```python
from build123d import *

# Parameters (mm, degrees)
EXTRUDE_1_DEPTH     = 64
SKETCH_2_W          = 73.114285432
SKETCH_2_H          = 69.176673978
SKETCH_2_R          = 31.5
CUT_EXTRUDE_2_DEPTH = 64
SKETCH_3_R          = 3.05
CUT_EXTRUDE_3_DEPTH = 64
SKETCH_4_R          = 1.55
CUT_EXTRUDE_4_DEPTH = 64


with BuildPart() as part:
    # 草图1 → 凸台-拉伸1 (new body)
    with BuildSketch(Plane(origin=(0, 0, 0), x_dir=(1, 0, 0), z_dir=(0, 1, 0))):
        with BuildLine():
            Line((-32, 0), (-7, 0))
            ThreePointArc((-7, 0), (-6.292893219, 0.292893219), (-6, 1))
            Line((-6, 1), (-6, 5))
            ThreePointArc((-6, 5), (-5.707106781, 5.707106781), (-5, 6))
            Line((-5, 6), (5, 6))
            ThreePointArc((5, 6), (5.707106781, 5.707106781), (6, 5))
            Line((6, 5), (6, 1))
            ThreePointArc((6, 1), (6.292893219, 0.292893219), (7, 0))
            Line((7, 0), (32, 0))
            Line((32, 0), (32, 2.5))
            Line((32, 2.5), (11, 2.5))
            ThreePointArc((11, 2.5), (10.292893219, 2.792893219), (10, 3.5))
            Line((10, 3.5), (10, 7.5))
            ThreePointArc((10, 7.5), (9.707106781, 8.207106781), (9, 8.5))
            Line((9, 8.5), (-9, 8.5))
            ThreePointArc((-9, 8.5), (-9.707106781, 8.207106781), (-10, 7.5))
            Line((-10, 7.5), (-10, 3.5))
            ThreePointArc((-10, 3.5), (-10.292893219, 2.792893219), (-11, 2.5))
            Line((-11, 2.5), (-32, 2.5))
            Line((-32, 2.5), (-32, 0))
        make_face()
    extrude(amount=EXTRUDE_1_DEPTH)

    # 草图2 → 切除-拉伸2 (cut)
    with BuildSketch(Plane.XY):
        with Locations((0, 32)):
            Rectangle(SKETCH_2_W, SKETCH_2_H)
        with Locations(Location((0, 32, 0), (0, 0, 290.438779576))):
            Circle(SKETCH_2_R, mode=Mode.SUBTRACT)
    extrude(amount=-CUT_EXTRUDE_2_DEPTH, mode=Mode.SUBTRACT)

    # 草图3 → 切除-拉伸3 (cut)
    with BuildSketch(Plane(origin=(0, 0, -2.5), x_dir=(-1, 0, 0), z_dir=(0, 0, -1))):
        with Locations((-17.67766953, 14.32233047)):
            Circle(SKETCH_3_R)
        with Locations((-17.67766953, 49.67766953)):
            Circle(SKETCH_3_R)
        with Locations((17.67766953, 49.67766953)):
            Circle(SKETCH_3_R)
        with Locations((17.67766953, 14.32233047)):
            Circle(SKETCH_3_R)
    extrude(amount=-CUT_EXTRUDE_3_DEPTH, mode=Mode.SUBTRACT)

    # 草图4 → 切除-拉伸4 (cut)
    with BuildSketch(Plane(origin=(0, 0, -8.5), x_dir=(-1, 0, 0), z_dir=(0, 0, -1))):
        with Locations((0, 54.5)):
            Circle(SKETCH_4_R)
        with Locations((0, 9.5)):
            Circle(SKETCH_4_R)
    extrude(amount=-CUT_EXTRUDE_4_DEPTH, mode=Mode.SUBTRACT)


solid = part.part
```
CAD build for the part. Positions are in the model's coordinates, mm. A direction names the side the tool comes from. Coordinates: 2 decimals unless noted, no trailing zeros. Order: outer loops, then holes, each group sorted by start corner. A loop starts at its lowest first (then second) coordinate and runs counter-clockwise, first axis right, second up. Notation, with made-up numbers: (29, -20) - (88, -20) arc R22 ccw to (88, 19) - close; hole circle Ø10 at (5.25, 63). An arc over 180 degrees is marked (long way). Use a Markdown table: item, result. Add a question column.
(1) Pull direction X, two halves, no side cores. Call faces 6 (the face through (-17.02, 46.7, -1.27)), 7 (the face through (-10, 32, -6)), 8 (the face through (-9.692, 61.972, -2.302)): +X half, -X half, draft (parallel to the pull), parting line (faces both ways), or undercut.
(2) Which spindle directions (+Z, -Z, +X, -X, +Y, -Y) get a long thin tool onto all of the face, cutting with end or side? Do faces 1 (the face through (6, 32, -3)), 2 (the face through (0, 32, -8.5)), 3 (the face through (10, 32, -5)), 4 (the face through (-19, 32, -2.5)), 5 (the face through (18.34, 46.7, -1.27)). Say none if no direction does.
(3) Drill centre lines: line 1 along Y through (x, z) = (0, -7.1); line 2 along X through (y, z) = (43, -5); line 3 along Y through (x, z) = (-18, -1.5). Where is each one in solid material? Low to high. Write a range as [from, to].
(4) Saw through at D-D (y = 9.5). Give the cut face in (x, z).
(5) Saw through at A-A (x = 0). Give the cut face in (y, z).
(6) Saw through at C-C (z = -6.75). Give the cut face in (x, y), then the cut area to 3 significant figures.
(7) Saw through at B-B (y = 32). Give the cut face in (x, z), then the cut area to 4 significant figures.
(8) Flat gauge pins, fed straight in: pin 1 (1.2 mm diameter, centred on y = 36, z = -3.5, fed in from -X); pin 2 (8 mm diameter, centred on x = -1.5, y = 23, fed in from +Z); pin 3 (2.5 mm diameter, centred on x = 0, y = 54.5, fed in from +Z); pin 4 (2 mm diameter, centred on y = 21, z = -6, fed in from +X). Where does each tip first touch, or does it go through?
Solved:
| question | item | result |
|---|---|---|
| 1 | face 6 | undercut |
| 1 | face 7 | -X half |
| 1 | face 8 | parting line |
| 2 | face 1 | +Z, +Y, -Y |
| 2 | face 2 | -Z, +X, -X, +Y, -Y |
| 2 | face 3 | -Z, +X, +Y, -Y |
| 2 | face 4 | -Z, -X, +Y, -Y |
| 2 | face 5 | +Z, -Z |
| 3 | line 1 | y = [0.5, 7.95], [11.05, 52.95], [56.05, 63.5] |
| 3 | line 2 | x = [-10, -6], [6, 10] |
| 3 | line 3 | y = [6.15, 11.29], [17.36, 46.64], [52.71, 57.85] |
| 4 | outline | (-22.05, -2.5) - (-11, -2.5) arc R1 cw to (-10, -3.5) - (-10, -7.5) arc R1 ccw to (-9, -8.5) - (-1.55, -8.5) - (-1.55, -6) - (-5, -6) arc R1 cw to (-6, -5) - (-6, -1) arc R1 ccw to (-7, 0) - (-22.05, 0) - close; (1.55, -8.5) - (9, -8.5) arc R1 ccw to (10, -7.5) - (10, -3.5) arc R1 cw to (11, -2.5) - (22.05, -2.5) - (22.05, 0) - (7, 0) arc R1 ccw to (6, -1) - (6, -5) arc R1 cw to (5, -6) - (1.55, -6) - close |
| 5 | outline | (0.5, -8.5) - (7.95, -8.5) - (7.95, -6) - (0.5, -6) - close; (11.05, -8.5) - (52.95, -8.5) - (52.95, -6) - (11.05, -6) - close; (56.05, -8.5) - (63.5, -8.5) - (63.5, -6) - (56.05, -6) - close |
| 6 | outline | (-10, 2.13) arc R31.5 ccw to (10, 2.13) - (10, 61.87) arc R31.5 ccw to (-10, 61.87) - close; hole circle Ø3.1 at (0, 9.5); hole circle Ø3.1 at (0, 54.5) |
| 6 | area | 1,220 mm² |
| 7 | outline | (-31.5, -2.5) - (-11, -2.5) arc R1 cw to (-10, -3.5) - (-10, -7.5) arc R1 ccw to (-9, -8.5) - (9, -8.5) arc R1 ccw to (10, -7.5) - (10, -3.5) arc R1 cw to (11, -2.5) - (31.5, -2.5) - (31.5, 0) - (7, 0) arc R1 ccw to (6, -1) - (6, -5) arc R1 cw to (5, -6) - (-5, -6) arc R1 cw to (-6, -5) - (-6, -1) arc R1 ccw to (-7, 0) - (-31.5, 0) - close |
| 7 | area | 205.5 mm² |
| 8 | pin 1 | stops at x = -10.2 |
| 8 | pin 2 | stops at z = -5.87 |
| 8 | pin 3 | passes through |
| 8 | pin 4 | stops at x = 10 |
